Autodesk Inventor part; units mm, degrees
ref_plane "YZ Plane" through (0, 0, 0) normal (1, 0, 0) x (0, 1, 0)
ref_plane "XZ Plane" through (0, 0, 0) normal (0, 1, 0) x (-1, 0, 0)
ref_plane "XY Plane" through (0, 0, 0) normal (0, 0, 1) x (1, 0, 0)
sketch "Sketch1" plane through (0, 0, 0) normal (0, 1, 0) x (-1, 0, 0)
  line L0 (0, 0) -> (3.5635, -2.0574)
  line L1 (0, 0) -> (4.1148, 0) construction
  line L2 (3.5635, -2.0574) -> (3.5635, -6.1722)
  line L3 (3.5635, -6.1722) -> (0, -8.2296)
  line L4 (0, -8.2296) -> (-3.5635, -6.1722)
  line L5 (-3.5635, -6.1722) -> (-3.5635, -2.0574)
  line L6 (-3.5635, -2.0574) -> (0, 0)
  dimension "d0" = 4.1148
  dimension "d1" = 30
  dimension "d2" = 4.1148
  dimension "d3" = 4.1148
  dimension "d4" = 120
extrude "Extrusion1" add sketch "Sketch1" along normal blind 3.429
sketch "Sketch2" plane through (0, 3.429, 0) normal (0, 1, 0) x (1, 0, 0)
  line L0 (-3.5635, 2.0574) -> (0, 0)
  line L1 (0, 0) -> (3.5635, 2.0574)
  line L2 (3.5635, 2.0574) -> (3.5635, 6.1722)
  line L3 (3.5635, 6.1722) -> (0, 8.2296)
  line L4 (0, 8.2296) -> (-3.5635, 6.1722)
  line L5 (-3.5635, 6.1722) -> (-3.5635, 2.0574)
  line L6 (0, 0) -> (0, 4.1148) construction
  circle A0 centre (0, 4.1148) radius 3.4036
  dimension "d8" = 6.8072
extrude "Extrusion2" add sketch "Sketch2" along normal blind 3.175 contours A0
hole "Hole1" at (0, 6.604, -4.1148) direction (0, -1, 0) diameter 5.334 end through all
thread "Thread1"
properties part number "HexCap"
Can you work these out from the model? Positions are in its coordinate system, mm. Give positions to 0.01 mm unless a question says otherwise; leave off trailing zeros. Loops run counter-clockwise (first coordinate to the right, second up) from the corner with the lowest first, then second, coordinate; pieces in that order, holes last. Notation, with made-up numbers: (24, 59.5) -> (61, 59.5) arc R23 ccw to (61, 69.5) -> close; hole circle Ø4 at (-39, 34). An arc over 180 degrees is marked (long way). Return JSON: item names as keys, results as strings.
Q1. I need wall thicknesses on probe 1 along X at (y, z) = (5.75, -4); probe 2 along Z at (x, y) = (0, 4.75); probe 3 along Z at (x, y) = (1.5, 6.25). Which ranges of each line are inside material? Lowest first, please.
Checks:
{"probe 1": "x = -3.4 to -2.66, 2.66 to 3.4", "probe 2": "z = -7.52 to -6.78, -1.45 to -0.71", "probe 3": "z = -7.17 to -6.32, -1.91 to -1.06"}
Q2. I want a section at D-D, the plane x = 3. List the corners of the cut face in (y, z) for me, then the cut area to 3 significant figures.
Checks:
{"outline": "(0, -6.5) -> (3.43, -6.5) -> (3.43, -5.72) -> (6.6, -5.72) -> (6.6, -2.51) -> (3.43, -2.51) -> (3.43, -1.73) -> (0, -1.73) -> close", "area": "26.5 mm2"}
Q3. We'd pull the mould along X, two halves only. Please class faces 1 (the face through (-0.8, 3.26, -1.57)), 2 (the face through (3.246, 4.994, -3.092)), 3 (the face through (-2, 6.604, -2)): released by +X, released by -X, zero draft, split by the parting line, or undercut.
Checks:
{"face 1": "undercut", "face 2": "split by the parting line", "face 3": "zero draft"}
Q4. I want a section at A-A, the plane y = 2.5. List the corners of the cut face in (x, z) for me.
Checks:
{"outline": "(-3.56, -6.17) -> (0, -8.23) -> (3.56, -6.17) -> (3.56, -2.06) -> (0, 0) -> (-3.56, -2.06) -> close; hole circle Ø5.33 at (0, -4.11)"}
Q5. I want a section at C-C, the plane z = -6.5. List the corners of the cut face in (x, y) for me, then the cut area to 3 significant figures.
Checks:
{"outline": "(-3, 0) -> (-1.19, 0) -> (-1.19, 6.6) -> (-2.43, 6.6) -> (-2.43, 3.43) -> (-3, 3.43) -> close; (1.19, 0) -> (3, 0) -> (3, 3.43) -> (2.43, 3.43) -> (2.43, 6.6) -> (1.19, 6.6) -> close", "area": "20.2 mm2"}
Q6. I want a section at B-B, the plane x = 1. List the corners of the cut face in (y, z) for me.
Checks:
{"outline": "(0, -7.65) -> (3.43, -7.65) -> (3.43, -7.37) -> (6.6, -7.37) -> (6.6, -6.59) -> (0, -6.59) -> close; (0, -1.64) -> (6.6, -1.64) -> (6.6, -0.86) -> (3.43, -0.86) -> (3.43, -0.58) -> (0, -0.58) -> close"}
Q7. For pin 1 Ø1 at (x, z) = (-1, -4) entering from -Y; pin 2 Ø3.5 at (x, z) = (0.5, -5.5) entering from +Y, each with a flat end and sliding along its axis, tell me the tip position at first contact or that it passes through.
Checks:
{"pin 1": "passes through", "pin 2": "stops at y = 6.6"}
